Check sheet for the modelled part. Datum: model origin and axes. Units: mm. A direction names the side the tool comes from. Round coordinates to 2 decimals unless told otherwise and drop trailing zeros. Order: outer loops, then holes, each group sorted by start corner. A loop starts at its lowest first (then second) coordinate and runs counter-clockwise, first axis right, second up.
Q1. Cross-section at B-B on x = 77.5. Record the cut outline in (y, z) (3 decimals).
Q2. Scan lines: probe 1 along X at (y, z) = (-26.5, 38.5) (3 decimals); probe 2 along X at (y, z) = (-21, 29.5) (3 decimals); probe 3 along Z at (x, y) = (-66.5, -22) (3 decimals). Record each from-to range of solid material in increasing order.
Q3. Cross-section at A-A on y = -23. Record the cut outline in (x, z) (3 decimals).
Q4. Depth check by flat-ended pin: P1, Ø9, axis at x = -79.5, y = -17.5, coming from the +Z side; P2, Ø5, axis at y = -16, z = 43.5, coming from the +X side (3 decimals); P3, Ø8, axis at x = 68.5, z = 38, coming from the +Y side; P4, Ø15, axis at x = 69.5, y = -16, coming from the +Z side (3 decimals). Enter the tip coordinate at first touch or a pass-through.
Q5. Cross-section at D-D on z = 46.5. Record the cut outline in (x, y) (3 decimals), then the cut area to 3 significant figures.
Q6. Cross-section at C-C on y = -11. Record the cut outline in (x, z) (3 decimals).
Q7. Set-up check for faces 1 (the flat face through (84, -15, 38.375)), 2 (the flat face through (-66, -15, 38.375)), 3 (the flat face through (-3, -30, 39)): record each of +Z, -Z, +X, -X, +Y, -Y from which the full face is reachable in a straight line by a thin tool's end or side.
from build123d import *

# Parameters (mm, degrees)
F1_DEPTH = 30
F4_DEPTH = 25
F5_DEPTH = 25


with BuildPart() as f1:
    # F0 (on Front) → F1 (new body)
    with BuildSketch(Plane.XZ):
        Polygon((-91.375001, 38.374996), (-91.375001, 28.374996), (88.624999, 28.374996), (88.624999, 38.374996), (58.624999, 38.374996), (58.624999, 48.374996), (-61.375001, 48.374996), (-61.375001, 38.374996), align=None)
    extrude(amount=F1_DEPTH)

    # F2 (on face) → F4 (cut)
    with BuildSketch(Plane.XY.offset(38.374996)):
        with BuildLine():
            ThreePointArc((73.624999, -25), (80.696067, -22.071068), (83.624999, -15))
            ThreePointArc((83.624999, -15), (80.696067, -7.928932), (73.624999, -5))
            ThreePointArc((73.624999, -5), (66.553931, -7.928932), (63.624999, -15))
            ThreePointArc((63.624999, -15), (66.553931, -22.071068), (73.624999, -25))
        make_face()
    extrude(amount=-F4_DEPTH, mode=Mode.SUBTRACT)

    # F3 (on face) → F5 (cut)
    with BuildSketch(Plane.XY.offset(38.374996)):
        with BuildLine():
            ThreePointArc((-76.375001, -25), (-69.303933, -22.071068), (-66.375001, -15))
            ThreePointArc((-66.375001, -15), (-69.303933, -7.928932), (-76.375001, -5))
            ThreePointArc((-76.375001, -5), (-83.446069, -7.928932), (-86.375001, -15))
            ThreePointArc((-86.375001, -15), (-83.446069, -22.071068), (-76.375001, -25))
        make_face()
    extrude(amount=-F5_DEPTH, mode=Mode.SUBTRACT)


solid = f1.part
Results found:
1. outline: (-30, 28.375) - (-24.219, 28.375) - (-24.219, 38.375) - (-30, 38.375) - close; (-5.781, 28.375) - (0, 28.375) - (0, 38.375) - (-5.781, 38.375) - close
2. probe 1: x = -61.375 to 58.625
2. probe 2: x = -91.375 to -84.375, -68.375 to 65.625, 81.625 to 88.625
2. probe 3: z = 28.375 to 38.375
3. outline: (-91.375, 28.375) - (-82.375, 28.375) - (-82.375, 38.375) - (-91.375, 38.375) - close; (-70.375, 28.375) - (67.625, 28.375) - (67.625, 38.375) - (58.625, 38.375) - (58.625, 48.375) - (-61.375, 48.375) - (-61.375, 38.375) - (-70.375, 38.375) - close; (79.625, 28.375) - (88.625, 28.375) - (88.625, 38.375) - (79.625, 38.375) - close
4. P1: passes through
4. P2: stops at x = 58.625
4. P3: stops at y = 0
4. P4: stops at z = 38.375
5. outline: (-61.375, -30) - (58.625, -30) - (58.625, 0) - (-61.375, 0) - close
5. area: 3,600 mm2
6. outline: (-91.375, 28.375) - (-85.54, 28.375) - (-85.54, 38.375) - (-91.375, 38.375) - close; (-67.21, 28.375) - (64.46, 28.375) - (64.46, 38.375) - (58.625, 38.375) - (58.625, 48.375) - (-61.375, 48.375) - (-61.375, 38.375) - (-67.21, 38.375) - close; (82.79, 28.375) - (88.625, 28.375) - (88.625, 38.375) - (82.79, 38.375) - close
7. face 1: +Z, +X, +Y, -Y
7. face 2: +Z, -X, +Y, -Y
7. face 3: +Z, -Z, +X, -X, -Y
